CAD build for the part. Positions are in the model's coordinates, mm. A direction names the side the tool comes from. Coordinates: 2 decimals unless noted, no trailing zeros. Order: outer loops, then holes, each group sorted by start corner. A loop starts at its lowest first (then second) coordinate and runs counter-clockwise, first axis right, second up. Notation, with made-up numbers: (4, 26.5) - (17, 26.5) arc R21 cw to (17, 54.5) - close; hole circle Ø4 at (69, 48). An arc over 180 degrees is marked (long way). Use one line per item in the form item = value.
```python
from build123d import *

# Parameters (mm, degrees)
F0_W     = 60
F0_H     = 54.918804
F1_DEPTH = 20
F2_DEPTH = 50


with BuildPart() as f1:
    # F0 (on Front) → F1 (new body)
    with BuildSketch(Plane.XZ):
        with Locations((-30, 27.459402)):
            Rectangle(F0_W, F0_H)
    extrude(amount=F1_DEPTH)

    # F0 (on Front) → F2 (join)
    with BuildSketch(Plane.XZ):
        Polygon((0, 54.918804), (0, 0), (20, 0), (20, 14.918804), (12, 14.918804), (12, 44.918804), (20, 44.918804), (20, 54.918804), align=None)
    extrude(amount=F2_DEPTH)


solid = f1.part
```
Item 1: Cut at B-B, the plane z = 12. Write the cut outline in (x, y).
Derived:
outline = (-60, -20) - (0, -20) - (0, -50) - (20, -50) - (20, 0) - (-60, 0) - close
Item 2: Cut at D-D, the plane x = -50. Write the cut outline in (y, z).
Derived:
outline = (-20, 0) - (0, 0) - (0, 54.92) - (-20, 54.92) - close
Item 3: Drop flat-ended pins along their axis: pin 1 (24 mm diameter, centred on y = -25, z = 27, fed in from +X); pin 2 (10 mm diameter, centred on x = -4, z = 18.5, fed in from +Y); pin 3 (12 mm diameter, centred on y = -35, z = 37.5, fed in from -X); pin 4 (16.5 mm diameter, centred on x = -34.5, z = 17, fed in from -Y). Give the stop position or say it passes through.
Derived:
pin_1 = 12
pin_2 = 0
pin_3 = 0
pin_4 = -20
Item 4: Two-plate mould, pull along Z, no slides. Class faces 4 (the face through (20, -25, 50)), 5 (the face through (-11, -14, 54.919)), 6 (the face through (16, -25, 44.919)): +Z half, -Z half, draft (parallel to the pull), parting line (faces both ways), or undercut.
Derived:
face_4 = draft
face_5 = +Z half
face_6 = undercut
Item 5: Cut at C-C, the plane y = -39. Write the cut outline in (x, z), plus the area to 3 significant figures.
Derived:
outline = (0, 0) - (20, 0) - (20, 14.92) - (12, 14.92) - (12, 44.92) - (20, 44.92) - (20, 54.92) - (0, 54.92) - close
area = 858 mm²
Item 6: Drill centre lines: line 1 (Y direction, x = -1.5, z = 43.5); line 2 (X direction, y = -30, z = 5); line 3 (Z direction, x = 16.5, y = -6.5). Where is each one in solid material? Low to high. Write a range as [from, to].
Derived:
line_1 = [-20, 0]
line_2 = [0, 20]
line_3 = [0, 14.92], [44.92, 54.92]
Item 7: Cut at A-A, the plane y = -14. Write the cut outline in (x, z), plus the area to 3 significant figures.
Derived:
outline = (-60, 0) - (20, 0) - (20, 14.92) - (12, 14.92) - (12, 44.92) - (20, 44.92) - (20, 54.92) - (-60, 54.92) - close
area = 4,150 mm²
Item 8: 3-axis set-ups, long thin cutter, end or side, ignore diameter. For faces 1 (the face through (0, -35, 28)), 2 (the face through (20, -25, 7)), 3 (the face through (12, -25, 30)): which of +Z, -Z, +X, -X, +Y, -Y reach the whole face in a straight line?
Derived:
face_1 = +Z, -Z, -X, -Y
face_2 = +Z, -Z, +X, +Y, -Y
face_3 = +X, +Y, -Y
